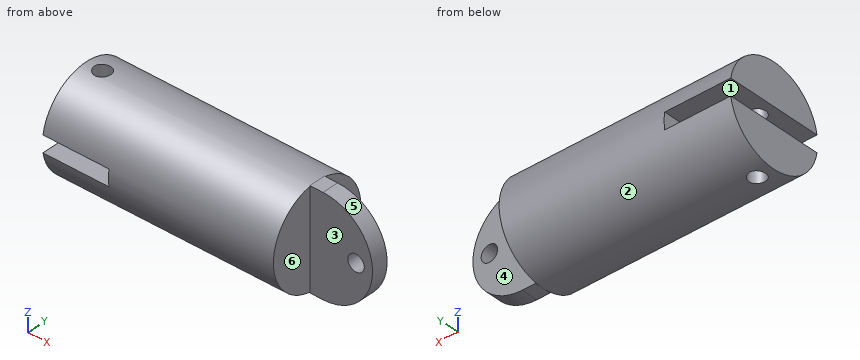
from build123d import *

# Parameters (mm, degrees)
SKETCH2_R               = 15
BOSS_EXTRUDE1_DEPTH     = 70
CUT_EXTRUDE1_DEPTH      = 74.143694192
CUT_EXTRUDE1_DEPTH_BACK = 74.143694192
SKETCH3_W               = 20
SKETCH3_H               = 5
CUT_EXTRUDE2_DEPTH      = 74.143694192
CUT_EXTRUDE2_DEPTH_BACK = 74.143694192
SKETCH6_R               = 2.5
SKETCH7_W               = 5
SKETCH7_H               = 30
BOSS_EXTRUDE2_DEPTH     = 4
BOSS_EXTRUDE3_DEPTH     = 5
CUT_EXTRUDE3_DEPTH      = 74.697015004
CUT_EXTRUDE3_DEPTH_BACK = 74.697015004
SKETCH9_R               = 2.5


with BuildPart() as part:
    # Sketch2 → Boss-Extrude1 (new body)
    with BuildSketch(Plane(origin=(0, 0, 0), x_dir=(0, 0, -1), z_dir=(1, 0, 0))):
        Circle(SKETCH2_R)
    extrude(amount=-BOSS_EXTRUDE1_DEPTH)

    # Sketch3 → Cut-Extrude1 (cut, two sides: drawn at the far end of the back side and taken through both)
    with BuildSketch(Plane(origin=(0, 0, 0), x_dir=(1, 0, 0), z_dir=(0, 1, 0)).offset(-CUT_EXTRUDE1_DEPTH_BACK)):
        with Locations((-60, 0)):
            Rectangle(SKETCH3_W, SKETCH3_H)
    extrude(amount=CUT_EXTRUDE1_DEPTH + CUT_EXTRUDE1_DEPTH_BACK, mode=Mode.SUBTRACT)

    # Sketch6 → Cut-Extrude2 (cut, two sides: drawn at the far end of the back side and taken through both)
    with BuildSketch(Plane.XY.offset(-CUT_EXTRUDE2_DEPTH_BACK)):
        with Locations((-65, 0)):
            Circle(SKETCH6_R)
    extrude(amount=CUT_EXTRUDE2_DEPTH + CUT_EXTRUDE2_DEPTH_BACK, mode=Mode.SUBTRACT)

    # Sketch7 → Boss-Extrude2 (add)
    with BuildSketch(Plane.YZ):
        Rectangle(SKETCH7_W, SKETCH7_H)
    extrude(amount=BOSS_EXTRUDE2_DEPTH)

    # Sketch8 → Boss-Extrude3 (add)
    with BuildSketch(Plane.XZ.offset(2.5)):
        with BuildLine():
            Line((4, 15), (4, -15))
            ThreePointArc((4, -15), (19, 0), (4, 15))
        make_face()
    extrude(amount=-BOSS_EXTRUDE3_DEPTH)

    # Sketch9 → Cut-Extrude3 (cut, two sides: drawn at the far end of the back side and taken through both)
    with BuildSketch(Plane.XZ.offset(2.5).offset(-CUT_EXTRUDE3_DEPTH_BACK)):
        with Locations(Location((14, 0, 0), (0, 0, 270))):
            Circle(SKETCH9_R)
    extrude(amount=CUT_EXTRUDE3_DEPTH + CUT_EXTRUDE3_DEPTH_BACK, mode=Mode.SUBTRACT)


solid = part.part
Model file for the job. Use its own axes, mm. Face numbers are marked on the shaded views. A direction names the side the tool comes from. Coordinates: 2 decimals unless noted, no trailing zeros. Loops run counter-clockwise (first coordinate to the right, second up) from the corner with the lowest first, then second, coordinate; pieces in that order, holes last. Notation, with made-up numbers: (-32.5, 85) -> (19.5, 85) arc R25 ccw to (19.5, 118) -> close; hole circle Ø11 at (74.25, 11). An arc over 180 degrees is marked (long way). Use one line per item in the form item = value. Start each with the question number.
(1) Cut at B-B on z = 12. Give the cut face in (x, y).
(2) Flat gauge pins, fed straight in: pin 1 (16 mm diameter, centred on x = -65, y = 0, fed in from -Z); pin 2 (9.5 mm diameter, centred on x = 7, z = -0.5, fed in from +Y); pin 3 (6 mm diameter, centred on x = -21, y = -12, fed in from -Z); pin 4 (4 mm diameter, centred on x = -43, y = 8, fed in from -Z). Where does each tip first touch, or does it go through?
(3) Pull direction Z, two halves, no side cores. Call the marked faces 1, 2 and 3: pulls with the +Z half, pulls with the -Z half, needs draft (parallel to the pull), parting line crosses it, or undercut.
(4) Cut at C-C on y = -9. Give the cut face in (x, z).
(5) Cut at A-A on x = -65. Give the cut face in (y, z).
(6) Probe probe 1 along X at (y, z) = (0.1, 0); probe 2 along X at (y, z) = (9, 3.5); probe 3 along X at (y, z) = (-10, 0). List the from-to ranges inside material, lowest first. Write a range as from..to.
(7) Tool access for the marked faces 4, 5 and 6: list every direction of +Z, -Z, +X, -X, +Y, -Y with a clear straight run to the whole face (end or side of a thin tool).
(8) Cut at D-D on x = 14. Give the cut face in (y, z).
Values:
q1.outline = (-70, -9) -> (0, -9) -> (0, -2.5) -> (13, -2.5) -> (13, 2.5) -> (0, 2.5) -> (0, 9) -> (-70, 9) -> close; hole circle Ø5 at (-65, 0)
q2.pin_1 = -15
q2.pin_2 = 2.5
q2.pin_3 = -12
q2.pin_4 = -13.75
q3.face_1 = undercut
q3.face_2 = parting line crosses it
q3.face_3 = needs draft
q4.outline = (-70, -12) -> (0, -12) -> (0, 12) -> (-70, 12) -> (-70, 2.5) -> (-50, 2.5) -> (-50, -2.5) -> (-70, -2.5) -> close
q5.outline = (-14.79, -2.5) arc R15 ccw to (-2.5, -14.79) -> (-2.5, -2.5) -> close; (-14.79, 2.5) -> (-2.5, 2.5) -> (-2.5, 14.79) arc R15 ccw to start; (2.5, -14.79) arc R15 ccw to (14.79, -2.5) -> (2.5, -2.5) -> close; (2.5, 2.5) -> (14.79, 2.5) arc R15 ccw to (2.5, 14.79) -> close
q6.probe_1 = -50..11.5, 16.5..19
q6.probe_2 = -70..0
q6.probe_3 = -50..0
q7.face_4 = +Z, -Z, +X, +Y
q7.face_5 = +X, +Y, -Y
q7.face_6 = +Z, -Z, +X, -Y
q8.outline = (-2.5, -11.18) -> (2.5, -11.18) -> (2.5, -2.5) -> (-2.5, -2.5) -> close; (-2.5, 2.5) -> (2.5, 2.5) -> (2.5, 11.18) -> (-2.5, 11.18) -> close
